Autodesk Inventor part; units mm, degrees
ref_plane "Work Plane2" through (-20.91, -9.18, -4.3) normal (0, 0, 1) x (1, 0, 0)
ref_plane "YZ Plane" through (0, 0, 0) normal (1, 0, 0) x (0, 1, 0)
ref_plane "XZ Plane" through (0, 0, 0) normal (0, 1, 0) x (-1, 0, 0)
ref_plane "Work Plane1" through (0, 0, 0) normal (0, 0, 1) x (1, 0, 0)
sketch "Sketch1" plane through (0, 0, 0) normal (0, 0, 1) x (1, 0, 0)
  line L0 (21.91, 12.18) -> (-21.91, 12.18)
  arc A0 (-23.91, -10.18) -> (-21.91, -12.18) centre (-21.91, -10.18) ccw
  line L1 (-21.91, -12.18) -> (21.91, -12.18)
  arc A1 (21.91, -12.18) -> (23.91, -10.18) centre (21.91, -10.18) ccw
  line L2 (23.91, -10.18) -> (23.91, -3.9)
  line L3 (23.91, -3.9) -> (22.39, -3.9)
  line L4 (22.39, -3.9) -> (22.39, -10.18)
  line L5 (22.39, -10.18) -> (-21.91, -10.18)
  line L6 (-21.91, -10.18) -> (-21.91, 10.18)
  line L7 (-21.91, 10.18) -> (22.39, 10.18)
  line L8 (22.39, 10.18) -> (22.39, 8.28)
  line L9 (22.39, 8.28) -> (23.91, 8.28)
  line L10 (23.91, 8.28) -> (23.91, 10.18)
  arc A2 (23.91, 10.18) -> (21.91, 12.18) centre (21.91, 10.18) ccw
  line L11 (21.91, 12.18) -> (-21.91, 12.18)
  arc A3 (-21.91, 12.18) -> (-23.91, 10.18) centre (-21.91, 10.18) ccw
  line L12 (-23.91, 10.18) -> (-23.91, -10.18)
  point P0 (0, 0)
extrude "Extrusion1" add sketch "Sketch1" along normal blind 2
sketch "Sketch2" plane through (22.39, 8.28, 0) normal (0, -1, 0) x (1, 0, 0)
  line L0 (0, 0) -> (1.52, 0)
  line L1 (1.52, 0) -> (1.52, 2)
  line L2 (0, 2) -> (1.52, 2)
  line L3 (0, 0) -> (0, 2)
  point P0 (-22.39, 0)
extrude "Extrusion2" add sketch "Sketch2" along normal up to next
sketch "Sketch4" plane through (-21.91, 10.18, 0) normal (0, -1, 0) x (1, 0, 0)
  line L0 (0, 0) -> (44.3, 0)
  line L1 (44.3, 0) -> (44.3, 2)
  line L2 (0, 2) -> (44.3, 2)
  line L3 (0, 0) -> (0, 2)
  point P0 (21.91, 0)
extrude "Extrusion3" add sketch "Sketch4" along normal up to next
fillet "Fillet1" radius 2 8 edges at (-23.3242, 11.5942, 2) (-23.91, 0, 2) (-23.3242, -11.5942, 2) (0, -12.18, 2) (23.3242, -11.5942, 2) (23.91, 0, 2) (23.3242, 11.5942, 2) (0, 12.18, 2)
ref_plane "Work Plane2" through (-20.91, -9.18, -4.3) normal (0, 0, 1) x (1, 0, 0)
sketch "Sketch3" plane through (0, 0, 0) normal (0, 0, 1) x (1, 0, 0)
  line L0 (-21.91, 10.18) -> (-19.41, 10.18)
  line L1 (-19.41, 7.68) -> (-19.41, 10.18)
  line L2 (-21.91, 7.68) -> (-19.41, 7.68)
  line L3 (-21.91, 7.68) -> (-21.91, 10.18)
  line L4 (19.89, 10.18) -> (22.39, 10.18)
  line L5 (19.89, 10.18) -> (19.89, 7.68)
  line L6 (19.89, 7.68) -> (22.39, 7.68)
  line L7 (22.39, 10.18) -> (22.39, 7.68)
  line L8 (-19.41, -10.18) -> (-21.91, -10.18)
  line L9 (-19.41, -10.18) -> (-19.41, -7.68)
  line L10 (-19.41, -7.68) -> (-21.91, -7.68)
  line L11 (-21.91, -10.18) -> (-21.91, -7.68)
  line L12 (22.39, -7.68) -> (22.39, -10.18)
  line L13 (22.39, -7.68) -> (19.89, -7.68)
  line L14 (19.89, -7.68) -> (19.89, -10.18)
  line L15 (22.39, -10.18) -> (19.89, -10.18)
  point P0 (0, 0)
extrude "Extrusion4" add sketch "Sketch3" against normal up to surface (4.3 mm away)
properties part number "NanoCaseTop"
Source: CAD feature listing. Evaluate the final solid. Frame: model axes, mm. A direction names the side the tool comes from. Give positions to 0.01 mm unless a question says otherwise; leave off trailing zeros. Loops run counter-clockwise (first coordinate to the right, second up) from the corner with the lowest first, then second, coordinate; pieces in that order, holes last. Notation, with made-up numbers: (44, 12) -> (101, 12) arc R30 cw to (101, 38) -> close; hole circle Ø5 at (-29, 0). An arc over 180 degrees is marked (long way). Use a Markdown table: item, result. Add a question column.
(1) Access query for faces 1 (the face through (-21, 7.68, -2)), 2 (the face through (-21.91, 9, -2)), 3 (the face through (21, 10.18, -2)), 4 (the face through (19.89, 9, -2)). Directions: +Z, -Z, +X, -X, +Y, -Y. A direction counts if a zero-diameter tool reaches every point of the face in a straight line with its end or side. Return the directions, or none.
(2) First-contact query: pin 1 Ø2 at (y, z) = (-8.5, -2.5) entering from +X; pin 2 Ø1.2 at (x, z) = (21, -2.5) entering from +Y; pin 3 Ø3 at (y, z) = (9, -2.5) entering from -X; pin 4 Ø3 at (x, z) = (-14, -3) entering from -Y. Flat tips, straight axial feed; report the tip coordinate or a pass-through.
(3) Section query A-A (z = -1.25). Output: boundary loops of the cut face in (x, y).
(4) Ray query, line 1 (Z direction, x = 22, y = 8.5); line 2 (Z direction, x = 6, y = -4.25); line 3 (Y direction, x = 1.5, z = 0.5). Return the intervals inside material, ascending.
(5) Pull-direction query (X, two-part tool) for faces 5 (the face through (21, -10.18, -2)), 6 (the face through (19.89, -9, -2)), 7 (the face through (22.39, -9, -2)); classes: +X half, -X half, draft (parallel to the pull), parting line (faces both ways), or undercut.
Checked values:
| question | item | result |
|---|---|---|
| 1 | face 1 | -Z, +X, -X |
| 1 | face 2 | -Z, -X, +Y, -Y |
| 1 | face 3 | -Z, +X, -X, +Y |
| 1 | face 4 | -Z, +Y, -Y |
| 2 | pin 1 | x = 22.39 |
| 2 | pin 2 | y = 10.18 |
| 2 | pin 3 | x = -21.91 |
| 2 | pin 4 | through |
| 3 | outline | (-21.91, -10.18) -> (-19.41, -10.18) -> (-19.41, -7.68) -> (-21.91, -7.68) -> close; (-21.91, 7.68) -> (-19.41, 7.68) -> (-19.41, 10.18) -> (-21.91, 10.18) -> close; (19.89, -10.18) -> (22.39, -10.18) -> (22.39, -7.68) -> (19.89, -7.68) -> close; (19.89, 7.68) -> (22.39, 7.68) -> (22.39, 10.18) -> (19.89, 10.18) -> close |
| 4 | line 1 | -4.3 to 2 |
| 4 | line 2 | 0 to 2 |
| 4 | line 3 | -12.12 to 12.12 |
| 5 | face 5 | draft |
| 5 | face 6 | undercut |
| 5 | face 7 | +X half |
